```python
from build123d import *

# Parameters (mm, degrees)
SKETCH1_R            = 10
MAIN_EXTRUSION_DEPTH = 6
SKETCH2_R            = 4
ID_BORE_DEPTH        = 20
SKETCH3_R            = 9
SKETCH3_R_2          = 5
SEAL_RECESS_DEPTH    = 5


with BuildPart() as part:
    # Sketch1 → main extrusion (new body)
    with BuildSketch(Plane(origin=(0, 0, 0), x_dir=(1, 0, 0), z_dir=(0, 1, 0))):
        with Locations(Location((0, 0, 0), (0, 0, 270))):
            Circle(SKETCH1_R)
    extrude(amount=MAIN_EXTRUSION_DEPTH)

    # Sketch2 → ID bore (cut)
    with BuildSketch(Plane(origin=(0, 6, 0), x_dir=(1, 0, 0), z_dir=(0, 1, 0))):
        with Locations(Location((0, 0, 0), (0, 0, 270))):
            Circle(SKETCH2_R)
    extrude(amount=-ID_BORE_DEPTH, mode=Mode.SUBTRACT)

    # Sketch3 → seal recess (cut)
    with BuildSketch(Plane(origin=(0, 6, 0), x_dir=(1, 0, 0), z_dir=(0, 1, 0))):
        with Locations(Location((0, 0, 0), (0, 0, 270))):
            Circle(SKETCH3_R)
        with Locations(Location((0, 0, 0), (0, 0, 270))):
            Circle(SKETCH3_R_2, mode=Mode.SUBTRACT)
    extrude(amount=-SEAL_RECESS_DEPTH, mode=Mode.SUBTRACT)


solid = part.part
```
Part model, mm, in its own coordinate system. A direction names the side the tool comes from. Round coordinates to 2 decimals unless told otherwise and drop trailing zeros. Write each loop counter-clockwise with the first axis right and the second up, starting at its lowest first coordinate (ties: lowest second). Pieces come first, ordered by that corner, then holes. Notation, with made-up numbers: (-8, 37.5) -> (18, 37.5) arc R18 ccw to (18, 65.5) -> close; hole circle Ø3 at (55.25, -16). An arc over 180 degrees is marked (long way). Return JSON: item names as keys, results as strings. Group by question number.
Q1. Mould opens along X. For faces 1 (the cylindrical face through (2.703, 3.535, 8.584)), 2 (the cylindrical face through (-9.76, 2.96, -2.17)), 3 (the flat face through (0.1, 0, 4.3)) say: pulls with the +X half, pulls with the -X half, needs draft (parallel to the pull), parting line crosses it, or undercut.
Q2. Saw through at A-A on z = 0. Write the cut outline in (x, y), plus the area to 3 significant figures.
Q3. Saw through at D-D on x = -6.5. Write the cut outline in (y, z).
Q4. Saw through at C-C on y = 4.05. Write the cut outline in (x, z), plus the area to 3 significant figures.
Q5. Probe L1, parallel to X at y = 2, z = 0; L2, parallel to Z at x = 1.75, y = 4.05; L3, parallel to Z at x = -0.75, y = 5.8. List the from-to ranges inside material, lowest first. Write a range as [from, to].
Q6. Saw through at B-B on x = 0. Write the cut outline in (y, z).
Q7. Which spindle directions (+Z, -Z, +X, -X, +Y, -Y) get a long thin tool onto all of the face, cutting with end or side? Do faces 4 (the flat face through (-4, 1, 4)), 5 (the flat face through (2, 6, -9)). Say none if no direction does.
Q8. Pin check, flat tips, straight feed: pin 1 (3 mm diameter, centred on x = 6.5, y = 2, fed in from -Z); pin 2 (2 mm diameter, centred on x = -5, y = 2, fed in from +Z). Stop position of each tip, or through.
Answer:
{
 "1": {"face 1": "undercut", "face 2": "parting line crosses it", "face 3": "needs draft"},
 "2": {"outline": "(-10, 0) -> (-4, 0) -> (-4, 6) -> (-5, 6) -> (-5, 1) -> (-9, 1) -> (-9, 6) -> (-10, 6) -> close; (4, 0) -> (10, 0) -> (10, 6) -> (9, 6) -> (9, 1) -> (5, 1) -> (5, 6) -> (4, 6) -> close", "area": "32.0 mm2"},
 "3": {"outline": "(0, -7.6) -> (6, -7.6) -> (6, -6.22) -> (1, -6.22) -> (1, 6.22) -> (6, 6.22) -> (6, 7.6) -> (0, 7.6) -> close"},
 "4": {"outline": "circle Ø20 at (0, 0); circle Ø10 at (0, 0); hole circle Ø18 at (0, 0); hole circle Ø8 at (0, 0)", "area": "88.0 mm2"},
 "5": {"L1": "[-10, -9], [-5, -4], [4, 5], [9, 10]", "L2": "[-9.85, -8.83], [-4.68, -3.6], [3.6, 4.68], [8.83, 9.85]", "L3": "[-9.97, -8.97], [-4.94, -3.93], [3.93, 4.94], [8.97, 9.97]"},
 "6": {"outline": "(0, -10) -> (6, -10) -> (6, -9) -> (1, -9) -> (1, -5) -> (6, -5) -> (6, -4) -> (0, -4) -> close; (0, 4) -> (6, 4) -> (6, 5) -> (1, 5) -> (1, 9) -> (6, 9) -> (6, 10) -> (0, 10) -> close"},
 "7": {"face 4": "+Y", "face 5": "+Z, -Z, +X, -X, +Y"},
 "8": {"pin 1": "z = -8.66", "pin 2": "z = 9.17"}
}
